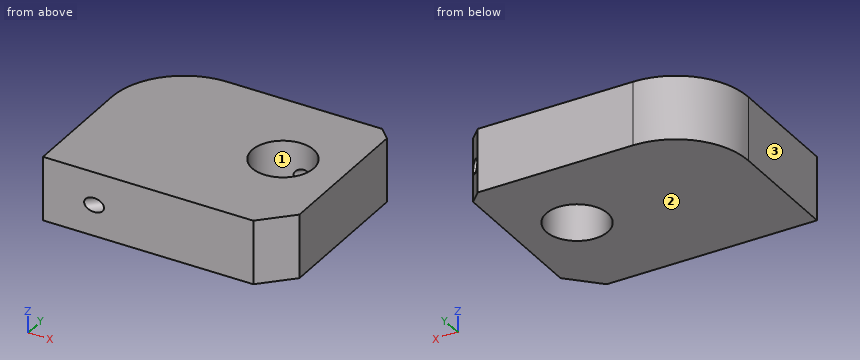
```python
from build123d import *

# Parameters (mm, degrees)
F0_R     = 5.385416
F1_DEPTH = 11.176
F2_SIZE  = 5.08
F3_SIZE  = 2
F4_R     = 1.230304
F5_DEPTH = 64.516


with BuildPart() as f1:
    # F0 (on Top) → F1 (new body)
    with BuildSketch(Plane.XY):
        with BuildLine():
            Line((-23.319686, 7.332434), (-23.319686, -13.010174))
            Line((-23.319686, -13.010174), (18.583678, -13.010174))
            Line((18.583678, -13.010174), (18.583678, 20.032434))
            Line((18.583678, 20.032434), (-10.619686, 20.032434))
            ThreePointArc((-10.619686, 20.032434), (-19.599942, 16.31269), (-23.319686, 7.332434))
        make_face()
        with Locations((8.170361, 4.813509)):
            Circle(F0_R, mode=Mode.SUBTRACT)
    extrude(amount=F1_DEPTH)

    # F2
    f2_edges = [f1.edges().sort_by_distance(p)[0] for p in [
        (18.583678, -13.010174, 5.588),
    ]]
    chamfer(f2_edges, length=F2_SIZE)

    # F3
    f3_edges = [f1.edges().sort_by_distance(p)[0] for p in [
        (18.583678, 20.032434, 5.588),
    ]]
    chamfer(f3_edges, length=F3_SIZE)

    # F4 (on face) → F5 (cut)
    with BuildSketch(Plane(origin=(18.308056, 18.308056, 0), x_dir=(-0.707107, 0.707107, 0), z_dir=(0.707107, 0.707107, 0))):
        with Locations((0.965202, 5.429061)):
            Circle(F4_R)
    extrude(amount=-F5_DEPTH, mode=Mode.SUBTRACT)


solid = f1.part
```
Design review of the part built by this model. Coordinates are the model's own, in mm. Face numbers are marked on the shaded views. Round coordinates to 2 decimals unless told otherwise and drop trailing zeros. Write each loop counter-clockwise with the first axis right and the second up, starting at its lowest first coordinate (ties: lowest second). Pieces come first, ordered by that corner, then holes.
Item 1: We need section D-D on z = 2. Write out the cut boundary in (x, y).
Item 2: For probe 1 along X at (y, z) = (2, 1); probe 2 along Y at (x, z) = (12.5, 7.5); probe 3 along Y at (x, z) = (-4, 5), list the stretches that pass through material, from the lowest coordinate up.
Item 3: We need section A-A on z = 4.75. Write out the cut boundary in (x, y).
Item 4: We need section B-B on x = 6. Write out the cut boundary in (y, z), and give its area (3 significant figures).
Item 5: The part is to be moulded in two halves that separate along X. For the marked faces 1, 2 and 3, say which applies: +X half, -X half, draft (parallel to the pull), parting line (faces both ways), or undercut.
Item 6: We need section C-C on y = 0. State how many separate pieces and enclosed holes the cut face has, and give its area (3 significant figures).
Returned:
1. outline: (-23.32, -13.01) - (13.5, -13.01) - (18.58, -7.93) - (18.58, 18.03) - (16.58, 20.03) - (-10.62, 20.03) arc R12.7 ccw to (-23.32, 7.33) - close; hole circle Ø10.77 at (8.17, 4.81)
2. probe 1: x = -23.32 to 3.58, 12.76 to 18.58
2. probe 2: y = -13.01 to 1.61, 8.02 to 20.03
2. probe 3: y = -13.01 to -4.27, -1 to 20.03
3. outline: (-23.32, -13.01) - (-15.83, -13.01) - (2.85, 5.67) arc R5.39 cw to (7.31, 10.13) - (16.9, 19.72) - (16.58, 20.03) - (-10.62, 20.03) arc R12.7 ccw to (-23.32, 7.33) - close; (-12.92, -13.01) - (13.5, -13.01) - (18.58, -7.93) - (18.58, 18.03) - (18.35, 18.27) - (9.97, 9.89) arc R5.39 cw (long way) to (3.1, 3.01) - close
4. outline: (-13.01, 0) - (-0.12, 0) - (-0.12, 11.18) - (-13.01, 11.18) - close; (9.74, 0) - (20.03, 0) - (20.03, 11.18) - (9.74, 11.18) - close
4. area: 259 mm2
5. face 1: undercut
5. face 2: draft
5. face 3: -X half
6. separate pieces: 2
6. enclosed holes: 1
6. area: 408 mm2
